Study the drawing (mm; zero at the part's minimum x, y, z) and answer. A direction names the side the tool comes from. Round coordinates to 2 decimals unless told otherwise and drop trailing zeros. Loops run counter-clockwise (first coordinate to the right, second up) from the corner with the lowest first, then second, coordinate; pieces in that order, holes last. Notation, with made-up numbers: M 38,77 L 70,77 A25 ccw 70,91 Z; hole C -29,-20 d4. An arc over 180 degrees is marked long. Put each result on its own line as item: value. Start each with the question number.
(1) Section A-A, the plane z = 13.25 is taken. Determine the outline of the cut face in (x, y).
(2) Section B-B, the plane x = 4.45 is taken. Determine the outline of the cut face in (y, z), then the cut area to 3 significant figures.
(3) Section C-C, the plane z = 9.5 is taken. Determine the outline of the cut face in (x, y), then the cut area to 3 significant figures.
(4) Which of the six approach directions +Z, -Z, +X, -X, +Y, -Y give full straight-line access (tool end or side, diameter ignored) to the marked faces 1, 2, 3, 4 and 5?
(5) Section D-D, the plane y = 15.75 is taken. Determine the outline of the cut face in (x, z), then the cut area to 3 significant figures.
(6) Straight lines are drawn through the part: line 1 (Z direction, x = 4.45, y = 20.1); line 2 (Z direction, x = 4.45, y = 17.75); line 3 (Z direction, x = 13.5, y = 6). For each, find the intervals that lie inside material, in ascending order.
(7) Flat-ended cylindrical pins translate along their axes: P1, Ø4, axis at x = 18.05, z = 13.25, coming from the +Y side; P2, Ø6.5, axis at y = 8, z = 6, coming from the -X side; P3, Ø1.5, axis at x = 4, y = 10, coming from the -Z side. Find the tip coordinate at first contact, or state that the pin passes through.
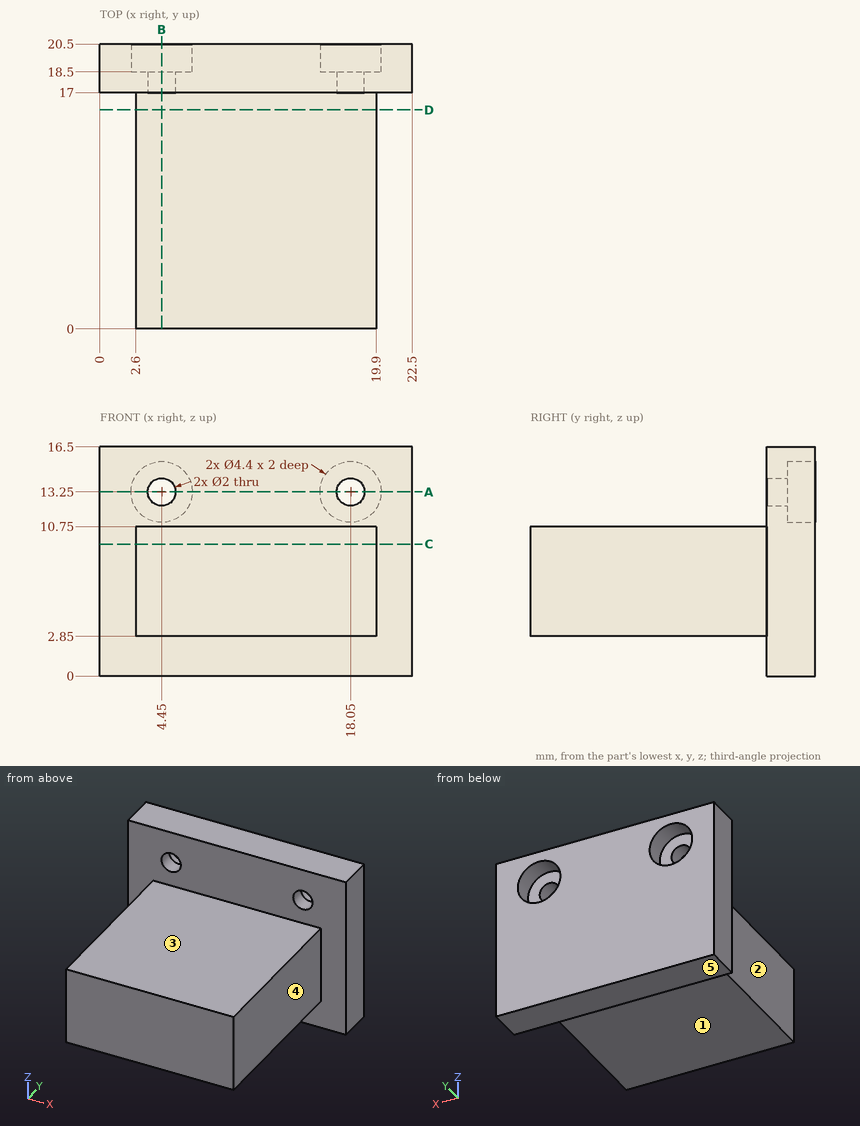
Recorded:
1. outline: M 0,17 L 3.45,17 L 3.45,18.5 L 2.25,18.5 L 2.25,20.5 L 0,20.5 Z; M 5.45,17 L 17.05,17 L 17.05,18.5 L 15.85,18.5 L 15.85,20.5 L 6.65,20.5 L 6.65,18.5 L 5.45,18.5 Z; M 19.05,17 L 22.5,17 L 22.5,20.5 L 20.25,20.5 L 20.25,18.5 L 19.05,18.5 Z
2. outline: M 0,2.85 L 17,2.85 L 17,0 L 20.5,0 L 20.5,11.05 L 18.5,11.05 L 18.5,12.25 L 17,12.25 L 17,10.75 L 0,10.75 Z; M 17,14.25 L 18.5,14.25 L 18.5,15.45 L 20.5,15.45 L 20.5,16.5 L 17,16.5 Z
2. area: 180 mm²
3. outline: M 0,17 L 2.6,17 L 2.6,0 L 19.9,0 L 19.9,17 L 22.5,17 L 22.5,20.5 L 0,20.5 Z
3. area: 373 mm²
4. face 1: -Z, +X, -X, -Y
4. face 2: +Z, -Z, -X, -Y
4. face 3: +Z, +X, -X, -Y
4. face 4: +Z, -Z, +X, -Y
4. face 5: -Z, +X, -X, +Y, -Y
5. outline: M 2.6,2.85 L 19.9,2.85 L 19.9,10.75 L 2.6,10.75 Z
5. area: 137 mm²
6. line 1: z = 0 to 11.05, 15.45 to 16.5
6. line 2: z = 0 to 12.25, 14.25 to 16.5
6. line 3: z = 2.85 to 10.75
7. P1: stops at y = 18.5
7. P2: stops at x = 2.6
7. P3: stops at z = 2.85
